Geometry: final body of the model. Coordinates: model frame, mm. A direction names the side the tool comes from. Give positions to 0.01 mm unless a question says otherwise; leave off trailing zeros. Write each loop counter-clockwise with the first axis right and the second up, starting at its lowest first coordinate (ties: lowest second). Pieces come first, ordered by that corner, then holes. Notation, with made-up numbers: (44.25, -2.5) -> (91.25, -2.5) arc R25 cw to (91.25, 32.5) -> close; hole circle Ø5 at (46.25, -9.75). An arc over 180 degrees is marked (long way). Answer in a Markdown table with one row per item. Add a question column.
Autodesk Inventor part; units mm, degrees
ref_plane "Work Plane1" through (0, 3.2, 0) normal (0, 1, 0) x (-1, 0, 0)
ref_plane "YZ Plane" through (0, 0, 0) normal (1, 0, 0) x (0, 1, 0)
ref_plane "XY Plane" through (0, 0, 0) normal (0, 0, 1) x (1, 0, 0)
sketch "Sketch1" plane through (0, 0, 0) normal (0, 0, 1) x (1, 0, 0)
  circle A0 centre (0, 0) radius 3.2
  dimension "d0" = 6.4
extrude "Extrusion1" add sketch "Sketch1" along normal blind 115
ref_plane "Work Plane1" through (0, 3.2, 0) normal (0, 1, 0) x (-1, 0, 0)
sketch "Sketch2" plane through (0, 3.2, 0) normal (0, 1, 0) x (-1, 0, 0)
  line L0 (0, -23) -> (0, 138)
  circle A0 centre (0, 107.5) radius 2.5
  line L1 (3.2, 115) -> (-3.2, 115)
  point P0 (0, 0)
  dimension "d11" = 5
  dimension "d12" = 7.5
extrude "Extrusion2" add sketch "Sketch2" along normal blind 4.25 and the other way blind 10.65
properties part number "Handle"
Q1. Section B-B on z = 107.5. Return loops of the section in (x, y), and give its area (3 significant figures).
Q2. Access query for faces 1 (the flat face through (0, 0, 115)), 2 (the cylindrical face through (-1.34, 4.76, 109.61)), 3 (the cylindrical face through (-2.385, -5.291, 108.251)). Directions: +Z, -Z, +X, -X, +Y, -Y. A direction counts if a zero-diameter tool reaches every point of the face in a straight line with its end or side. Return the directions, or none.
Q3. Line query: probe 1 along X at (y, z) = (-2, 105.5); probe 2 along Z at (x, y) = (0, 4). Output: solid intervals per line, ascending. Write a range as from..to.
Q4. Section D-D on z = 36. Return loops of the section in (x, y), and give its area (3 significant figures).
Q5. Section C-C on y = 4.5. Return loops of the section in (x, z).
Q6. Contact query for a flat-ended pin moving along its axis: pin 1 Ø6 at (y, z) = (3.5, 94) entering from -X. Output: stop coordinate, or through.
Q7. Section A-A on x = 0. Return loops of the section in (y, z).
Checks:
| question | item | result |
|---|---|---|
| 1 | outline | (-2.5, -7.45) -> (2.5, -7.45) -> (2.5, -2) arc R3.2 ccw to (2.5, 2) -> (2.5, 7.45) -> (-2.5, 7.45) -> (-2.5, 2) arc R3.2 ccw to (-2.5, -2) -> close |
| 1 | area | 78.3 mm^2 |
| 2 | face 1 | +Z, +X, -X, +Y, -Y |
| 2 | face 2 | +Y |
| 2 | face 3 | -Y |
| 3 | probe 1 | -2.5..2.5 |
| 3 | probe 2 | 105..110 |
| 4 | outline | circle Ø6.4 at (0, 0) |
| 4 | area | 32.2 mm^2 |
| 5 | outline | circle Ø5 at (0, 107.5) |
| 6 | pin 1 | x = -3.16 |
| 7 | outline | (-7.45, 105) -> (-3.2, 105) -> (-3.2, 0) -> (3.2, 0) -> (3.2, 105) -> (7.45, 105) -> (7.45, 110) -> (3.2, 110) -> (3.2, 115) -> (-3.2, 115) -> (-3.2, 110) -> (-7.45, 110) -> close |
